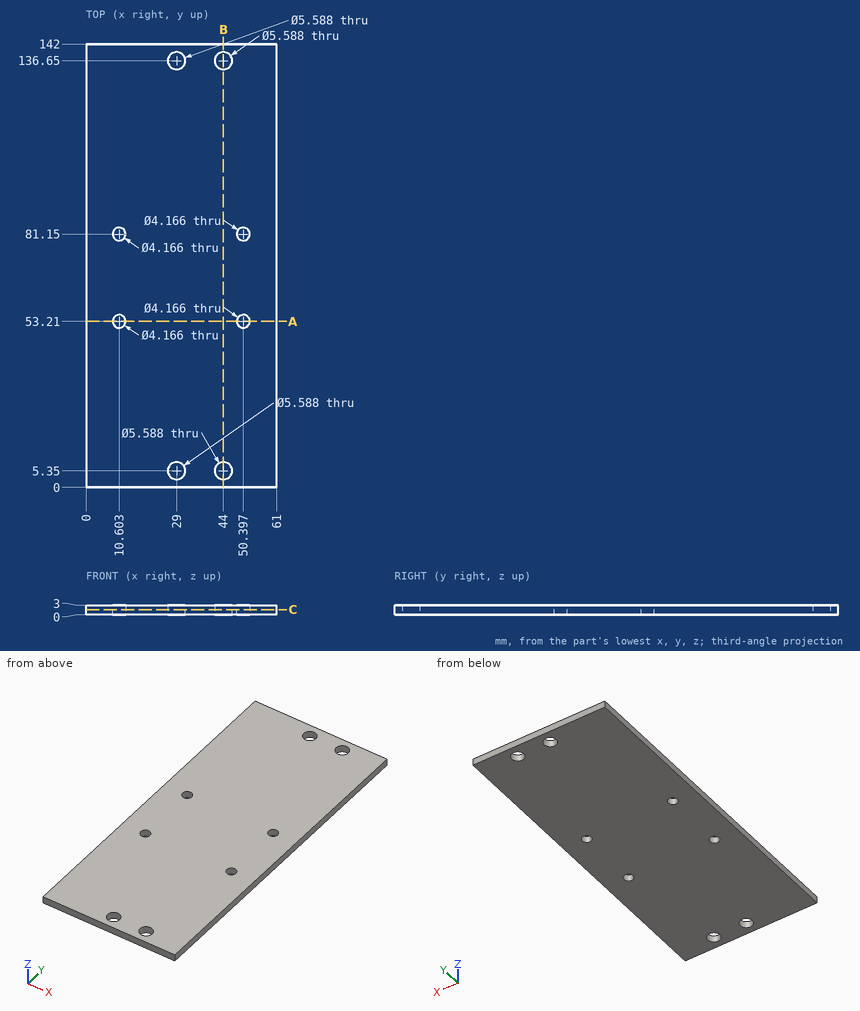
Geometry check sheet. Reference: drawing and pictorial views, mm from the part's lowest x, y, z. Coordinates: 2 decimals unless noted, no trailing zeros. Loops run counter-clockwise (first coordinate to the right, second up) from the corner with the lowest first, then second, coordinate; pieces in that order, holes last.
1) Sectioned sample at B-B (x = 44). Record the boundary of the cut face in (y, z).
2) Sectioned sample at A-A (y = 53.21). Record the boundary of the cut face in (x, z).
3) Sectioned sample at C-C (z = 1.65). Count the separate pieces of the cut face and the enclosed holes in it, and give its area (3 significant figures).
4) Gauge pin test, flat end, axial feed: pin 1 (3.5 mm diameter, centred on x = 44, y = 5.35, fed in from -Z). Record the tip position at first contact, or that the pin passes through.
5) Material ranges on probe 1 along X at (y, z) = (81, 1) (1 decimal); probe 2 along Y at (x, z) = (9.5, 1.05) (1 decimal); probe 3 along Y at (x, z) = (49, 2.4) (1 decimal), recorded low to high.
Check sheet entries:
1. outline: (0, 0) - (2.56, 0) - (2.56, 3) - (0, 3) - close; (8.14, 0) - (133.86, 0) - (133.86, 3) - (8.14, 3) - close; (139.44, 0) - (142, 0) - (142, 3) - (139.44, 3) - close
2. outline: (0, 0) - (8.52, 0) - (8.52, 3) - (0, 3) - close; (12.69, 0) - (48.31, 0) - (48.31, 3) - (12.69, 3) - close; (52.48, 0) - (61, 0) - (61, 3) - (52.48, 3) - close
3. separate pieces: 1
3. enclosed holes: 8
3. area: 8,510 mm2
4. pin 1: passes through
5. probe 1: x = 0 to 8.5, 12.7 to 48.3, 52.5 to 61
5. probe 2: y = 0 to 51.4, 55 to 79.4, 82.9 to 142
5. probe 3: y = 0 to 51.7, 54.8 to 79.6, 82.7 to 142
